Here's how the part is built. I have some questions about the finished solid (model axes, mm). A direction names the side the tool comes from. Give positions to 0.01 mm unless a question says otherwise; leave off trailing zeros. Write each loop counter-clockwise with the first axis right and the second up, starting at its lowest first coordinate (ties: lowest second). Pieces come first, ordered by that corner, then holes. Notation, with made-up numbers: (-0.5, -16.75) - (10.5, -16.75) arc R19 cw to (10.5, 13.25) - close; hole circle Ø10 at (79, -1.75). An arc over 180 degrees is marked (long way). Use a Markdown table: item, result.
```python
from build123d import *

# Parameters (mm, degrees)
F2_W    = 0.65
F2_H    = 1
F4_R    = 0.2
F5_SIZE = 0.2


with BuildPart() as f1:
    # F0 (on Front) → F1 (revolve)
    with BuildSketch(Plane.XZ):
        Polygon((0, -27), (0, 27), (-6, 27), (-6, 17), (-7, 17), (-7, -17), (-6, -17), (-6, -27), align=None)
    revolve(axis=Axis((0, 0, -1.756099), (0, 0, -1)))

    # F2 (on Front) → F3 (revolve, cut)
    with BuildSketch(Plane.XZ):
        with Locations((-5.675, 25.7)):
            Rectangle(F2_W, F2_H)
        with Locations((-5.675, -25.7)):
            Rectangle(F2_W, F2_H)
    revolve(axis=Axis((0, 0, 0.721304), (0, 0, -1)), mode=Mode.SUBTRACT)

    # F4
    f4_edges = [f1.edges().sort_by_distance(p)[0] for p in [
        (6, 0, 17),
        (6, 0, -17),
    ]]
    fillet(f4_edges, radius=F4_R)

    # F5
    f5_edges = [f1.edges().sort_by_distance(p)[0] for p in [
        (7, 0, -17),
        (7, 0, 17),
        (6, 0, 27),
        (6, 0, -27),
    ]]
    chamfer(f5_edges, length=F5_SIZE)


solid = f1.part
```
Item 1: For faces 1 (the cylindrical face through (6, 0, -21)), 2 (the flat face through (0, 0, 27)), 3 (the cylindrical face through (5.994, 0.264, 26.496)), which set-ups out of +Z, -Z, +X, -X, +Y, -Y let a thin tool reach every point of the face, with its end or its side?
Values:
| item | result |
|---|---|
| face 1 | -Z |
| face 2 | +Z, +X, -X, +Y, -Y |
| face 3 | +Z |
Item 2: If we section it at B-B, the plane z = -7: Write out the boundary of the cut face in (x, y), plus the area to 3 significant figures.
Values:
| item | result |
|---|---|
| outline | circle Ø14 at (0, 0) |
| area | 154 mm2 |
Item 3: Will this pin go through, and if not, where does the flat tip stop? pin 1 Ø6 at (x, z) = (5, -2.5) entering from -Y.
Values:
| item | result |
|---|---|
| pin 1 | stops at y = -6.71 |
Item 4: Thinking about a two-plate mould opening in Z: for faces 4 (the cylindrical face through (1.16, -5.223, 25.707)), 5 (the flat face through (0, 0, -27)), 6 (the cylindrical face through (5.994, 0.264, -26.504)), 7 (the cylindrical face through (1.16, -5.223, -25.693)), which applies, +Z half, -Z half, draft (parallel to the pull), parting line (faces both ways), or undercut?
Values:
| item | result |
|---|---|
| face 4 | undercut |
| face 5 | -Z half |
| face 6 | draft |
| face 7 | undercut |
Item 5: I need wall thicknesses on line 1 along Z through (x, y) = (-5.5, 0.75); line 2 along Z through (x, y) = (-2.5, -6); line 3 along Y through (x, z) = (-3.25, 5.5). Which ranges of each line are inside material? Lowest first, please. Write a range as [from, to].
Values:
| item | result |
|---|---|
| line 1 | z = [-27, -26.2], [-25.2, 25.2], [26.2, 27] |
| line 2 | z = [-17, 17] |
| line 3 | y = [-6.2, 6.2] |
Item 6: If we section it at A-A, the plane z = -22: Write out the boundary of the cut face in (x, y).
Values:
| item | result |
|---|---|
| outline | circle Ø12 at (0, 0) |
